The model under review builds one solid part; all positions refer to its coordinate system, in mm. Face numbers are marked on the shaded views. A direction names the side the tool comes from. Round coordinates to 2 decimals unless told otherwise and drop trailing zeros. Order: outer loops, then holes, each group sorted by start corner. A loop starts at its lowest first (then second) coordinate and runs counter-clockwise, first axis right, second up. Notation, with made-up numbers: M 24.5,66 L 31.5,66 A27 ccw 31.5,97 Z; hole C 15,88 d11. An arc over 180 degrees is marked long. Answer as a JSON object with one key per item and string values. Group by question number.
1) Consider section B-B, the plane y = -5. Write out the cut boundary in (x, z), then the cut area to 3 significant figures.
2) To check wall thickness, follow line 1 (Y direction, x = 2, z = 3); line 2 (X direction, y = 3.5, z = 0.25); line 3 (Z direction, x = -3, y = 12). State the ranges of each line that lie inside material, in increasing order.
3) The part is to be moulded in two halves that separate along Y. For the marked faces 6, 7, 8 and 9, say which applies: +Y half, -Y half, draft (parallel to the pull), parting line (faces both ways), or undercut.
4) Consider section A-A, the plane z = 2.75. Write out the cut boundary in (x, y).
5) For the marked faces 1, 2, 3, 4 and 5, list the 3-axis set-ups (+Z, -Z, +X, -X, +Y, -Y) from which the entire face can be reached by the end or side of a thin tool; tool diameter is ignored.
6) Insertion check: pin 1 Ø3 at (x, z) = (-10.5, -3.5) entering from -Y; pin 2 Ø10 at (x, z) = (0.5, -0.5) entering from -Y; pin 3 Ø8 at (x, z) = (1.5, -6) entering from +Y; pin 4 Ø13 at (x, y) = (-3.5, 6.5) entering from +Z. Each pin has a flat end and moves straight along its axis. Give the tip position at first contact, or say it passes through.
7) Consider section C-C, the plane x = 4. Write out the cut boundary in (y, z).
8) Consider section D-D, the plane z = -3.75. Write out the cut boundary in (x, y).
```python
from build123d import *

# Parameters (mm, degrees)
BOSS_EXTRUDE1_DEPTH = 5
FILLET3_R           = 1
BOSS_EXTRUDE2_DEPTH = 13.6


with BuildPart() as part:
    # Sketch1 → Boss-Extrude1 (new body)
    with BuildSketch(Plane.XY):
        with BuildLine():
            Line((-12.15, -16.65), (12.15, -16.65))
            ThreePointArc((12.15, -16.65), (14.271320344, -15.771320344), (15.15, -13.65))
            Line((15.15, -13.65), (15.15, 13.65))
            ThreePointArc((15.15, 13.65), (14.271320344, 15.771320344), (12.15, 16.65))
            Line((12.15, 16.65), (-12.15, 16.65))
            ThreePointArc((-12.15, 16.65), (-14.271320344, 15.771320344), (-15.15, 13.65))
            Line((-15.15, 13.65), (-15.15, -13.65))
            ThreePointArc((-15.15, -13.65), (-14.271320344, -15.771320344), (-12.15, -16.65))
        make_face()
        with BuildLine():
            Line((-5.524448559, 13.45), (5.524448559, 13.45))
            ThreePointArc((5.524448559, 13.45), (6.452181075, 13.302948016), (7.288963652, 12.876208253))
            Line((7.288963652, 12.876208253), (10.764515093, 10.348534478))
            ThreePointArc((10.764515093, 10.348534478), (11.673344841, 9.28365916), (12, 7.922326225))
            Line((12, 7.922326225), (12, 0.45))
            ThreePointArc((12, 0.45), (11.121320344, -1.671320344), (9, -2.55))
            Line((9, -2.55), (-9, -2.55))
            ThreePointArc((-9, -2.55), (-11.121320344, -1.671320344), (-12, 0.45))
            Line((-12, 0.45), (-12, 7.922326225))
            ThreePointArc((-12, 7.922326225), (-11.673344841, 9.28365916), (-10.764515093, 10.348534478))
            Line((-10.764515093, 10.348534478), (-7.288963652, 12.876208253))
            ThreePointArc((-7.288963652, 12.876208253), (-6.452181075, 13.302948016), (-5.524448559, 13.45))
        make_face(mode=Mode.SUBTRACT)
        with BuildLine():
            Line((-12, -6.65), (-12, -11.65))
            ThreePointArc((-12, -11.65), (-11.707106781, -12.357106781), (-11, -12.65))
            Line((-11, -12.65), (11, -12.65))
            ThreePointArc((11, -12.65), (11.707106781, -12.357106781), (12, -11.65))
            Line((12, -11.65), (12, -6.65))
            ThreePointArc((12, -6.65), (11.707106781, -5.942893219), (11, -5.65))
            Line((11, -5.65), (-11, -5.65))
            ThreePointArc((-11, -5.65), (-11.707106781, -5.942893219), (-12, -6.65))
        make_face(mode=Mode.SUBTRACT)
    extrude(amount=BOSS_EXTRUDE1_DEPTH)

    # Fillet3
    fillet3_edges = [part.edges().sort_by_distance(p)[0] for p in [
        (-14.271320344, 15.771320344, 5),
        (-15.15, 0, 5),
        (-14.271320344, -15.771320344, 5),
        (0, -16.65, 5),
        (14.271320344, -15.771320344, 5),
        (15.15, 0, 5),
        (14.271320344, 15.771320344, 5),
        (0, 16.65, 5),
    ]]
    fillet(fillet3_edges, radius=FILLET3_R)

    # Sketch3 → Boss-Extrude2 (add)
    with BuildSketch(Plane(origin=(0, 0, 0), x_dir=(-1, 0, 0), z_dir=(0, 0, -1))):
        with BuildLine():
            Line((-13.5, 14.15), (-13.5, -14.15))
            ThreePointArc((-13.5, -14.15), (-13.104594155, -15.104594155), (-12.15, -15.5))
            Line((-12.15, -15.5), (12.15, -15.5))
            ThreePointArc((12.15, -15.5), (13.104594155, -15.104594155), (13.5, -14.15))
            Line((13.5, -14.15), (13.5, 14.15))
            ThreePointArc((13.5, 14.15), (13.104594155, 15.104594155), (12.15, 15.5))
            Line((12.15, 15.5), (-12.15, 15.5))
            ThreePointArc((-12.15, 15.5), (-13.104594155, 15.104594155), (-13.5, 14.15))
        make_face()
    extrude(amount=BOSS_EXTRUDE2_DEPTH)


solid = part.part
```
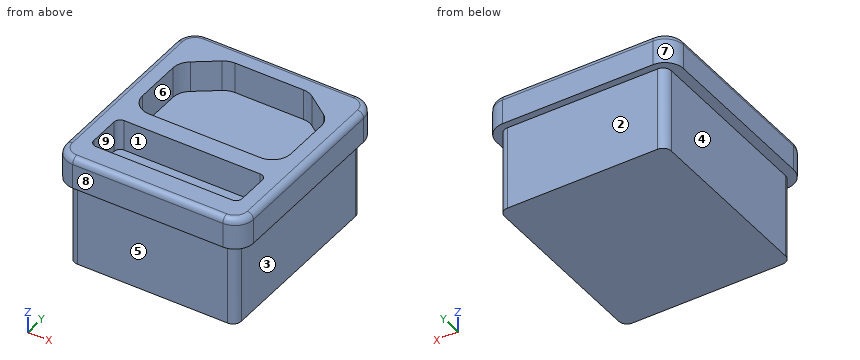
Results list:
{
 "1": {"outline": "M -15.15,0 L -13.5,0 L -13.5,-13.6 L 13.5,-13.6 L 13.5,0 L 15.15,0 L 15.15,4 A1 ccw 14.15,5 L -14.15,5 A1 ccw -15.15,4 Z", "area": "518 mm^2"},
 "2": {"line 1": "-16.65 to -12.65, -5.65 to -2.55, 13.45 to 16.65", "line 2": "-15.15 to -12, 12 to 15.15", "line 3": "-13.6 to 0"},
 "3": {"face 6": "undercut", "face 7": "+Y half", "face 8": "-Y half", "face 9": "undercut"},
 "4": {"outline": "M -15.15,-13.65 A3 ccw -12.15,-16.65 L 12.15,-16.65 A3 ccw 15.15,-13.65 L 15.15,13.65 A3 ccw 12.15,16.65 L -12.15,16.65 A3 ccw -15.15,13.65 Z; hole M -12,-11.65 A1 ccw -11,-12.65 L 11,-12.65 A1 ccw 12,-11.65 L 12,-6.65 A1 ccw 11,-5.65 L -11,-5.65 A1 ccw -12,-6.65 Z; hole M -12,0.45 A3 ccw -9,-2.55 L 9,-2.55 A3 ccw 12,0.45 L 12,7.92 A3 ccw 10.76,10.35 L 7.29,12.88 A3 ccw 5.52,13.45 L -5.52,13.45 A3 ccw -7.29,12.88 L -10.76,10.35 A3 ccw -12,7.92 Z"},
 "5": {"face 1": "+Z", "face 2": "-Z, +X, -X, +Y", "face 3": "-Z, +X, +Y, -Y", "face 4": "-Z, -X, +Y, -Y", "face 5": "-Z, +X, -X, -Y"},
 "6": {"pin 1": "y = -15.5", "pin 2": "y = -16.65", "pin 3": "y = 15.5", "pin 4": "z = 0"},
 "7": {"outline": "M -16.65,0 L -15.5,0 L -15.5,-13.6 L 15.5,-13.6 L 15.5,0 L 16.65,0 L 16.65,4 A1 ccw 15.65,5 L 13.45,5 L 13.45,0 L -2.55,0 L -2.55,5 L -5.65,5 L -5.65,0 L -12.65,0 L -12.65,5 L -15.65,5 A1 ccw -16.65,4 Z"},
 "8": {"outline": "M -13.5,-14.15 A1.35 ccw -12.15,-15.5 L 12.15,-15.5 A1.35 ccw 13.5,-14.15 L 13.5,14.15 A1.35 ccw 12.15,15.5 L -12.15,15.5 A1.35 ccw -13.5,14.15 Z"}
}
